For this review, use the dimensioned drawing (mm, ordinates from the lowest corner) and the shaded views. A direction names the side the tool comes from. Round coordinates to 2 decimals unless told otherwise and drop trailing zeros. Loops run counter-clockwise (first coordinate to the right, second up) from the corner with the lowest first, then second, coordinate; pieces in that order, holes last. Notation, with made-up numbers: M 82.5,41.5 L 137.5,41.5 A22 ccw 137.5,53.5 Z; hole C 40.25,47.25 d1. An arc over 180 degrees is marked long. Answer as a JSON object with one key per item and string values. Group by question number.
Item 1: The part is to be moulded in two halves that separate along Z. For the marked faces 3, 4, 5 and 6, say which applies: +Z half, -Z half, draft (parallel to the pull), parting line (faces both ways), or undercut.
Item 2: To check wall thickness, follow line 1 (Y direction, x = 12.7, z = 9.5); line 2 (X direction, y = 68.5, z = 7) (1 decimal); line 3 (X direction, y = 12, z = 4). State the ranges of each line that lie inside material, in increasing order.
Item 3: Consider section D-D (z = 41). Give the boundary of the cut face in (x, y).
Item 4: Consider section B-B (x = 12.7). Give the boundary of the cut face in (y, z), and give its area (3 significant figures).
Item 5: Tool access review of the marked faces 1 and 2: name each direction out of +Z, -Z, +X, -X, +Y, -Y from which nothing blocks a thin tool from reaching the whole face with its end or side.
Item 6: Consider section A-A (z = 4.5). Give the boundary of the cut face in (x, y), and give its area (3 significant figures).
Item 7: Consider section C-C (x = 130). Give the boundary of the cut face in (y, z), and give its area (3 significant figures).
Item 8: Insertion check: P1, Ø10, axis at x = 133.35, y = 12.7, coming from the +Z side; P2, Ø5, axis at x = 17.5, y = 17, coming from the +Z side; P3, Ø3, axis at x = 131, z = 14, coming from the +Y side; P4, Ø1.5, axis at y = 28.5, z = 33.5, coming from the -X side (3 decimals). Each pin has a flat end and moves straight along its axis. Give the tip position at first contact, or say it passes through.
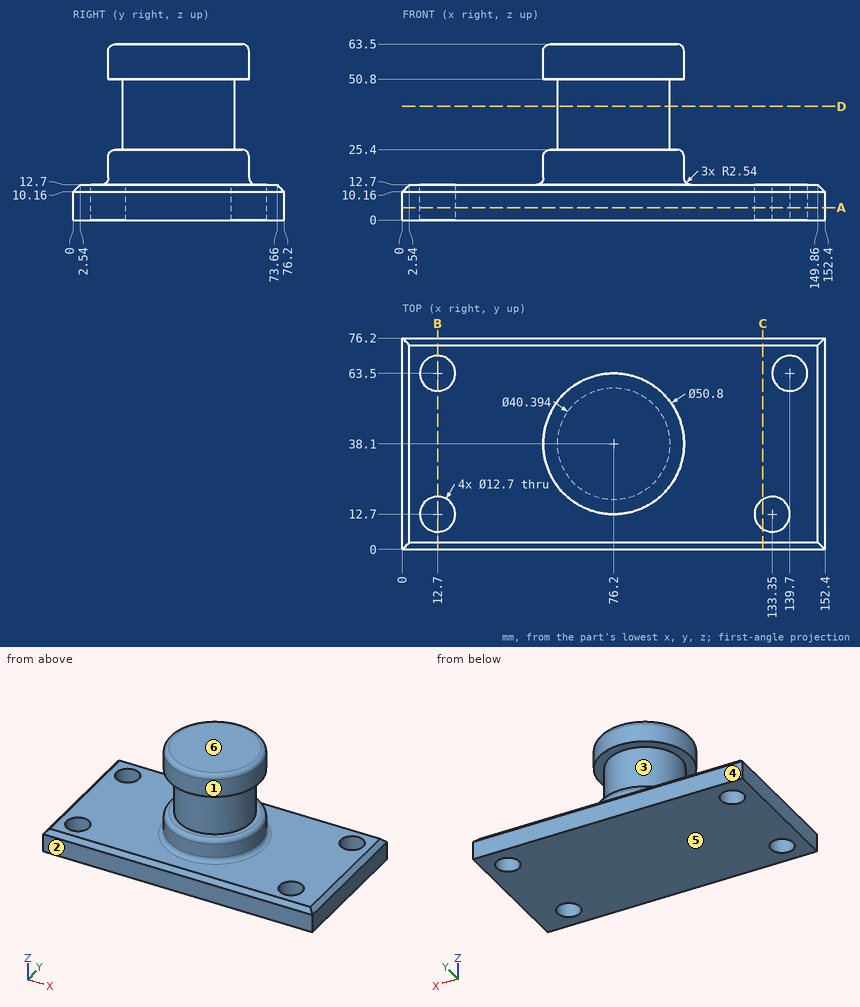
Geometry results:
{
 "1": {"face 3": "undercut", "face 4": "draft", "face 5": "-Z half", "face 6": "+Z half"},
 "2": {"line 1": "y = 0 to 6.35, 19.05 to 57.15, 69.85 to 76.2", "line 2": "x = 0 to 8.8, 16.6 to 135.8, 143.6 to 152.4", "line 3": "x = 0 to 6.39, 19.01 to 127.04, 139.66 to 152.4"},
 "3": {"outline": "C 76.2,38.1 d40.39"},
 "4": {"outline": "M 0,0 L 6.35,0 L 6.35,12.7 L 2.54,12.7 L 0,10.16 Z; M 19.05,0 L 57.15,0 L 57.15,12.7 L 19.05,12.7 Z; M 69.85,0 L 76.2,0 L 76.2,10.16 L 73.66,12.7 L 69.85,12.7 Z", "area": "639 mm^2"},
 "5": {"face 1": "+Z", "face 2": "+Z, -Z, +X, -X, -Y"},
 "6": {"outline": "M 0,0 L 152.4,0 L 152.4,76.2 L 0,76.2 Z; hole C 12.7,12.7 d12.7; hole C 12.7,63.5 d12.7; hole C 133.35,12.7 d12.7; hole C 139.7,63.5 d12.7", "area": "11,100 mm^2"},
 "7": {"outline": "M 0,0 L 7.31,0 L 7.31,12.7 L 2.54,12.7 L 0,10.16 Z; M 18.09,0 L 76.2,0 L 76.2,10.16 L 73.66,12.7 L 18.09,12.7 Z", "area": "824 mm^2"},
 "8": {"P1": "passes through", "P2": "stops at z = 12.7", "P3": "stops at y = 73.86", "P4": "stops at x = 58.045"}
}
